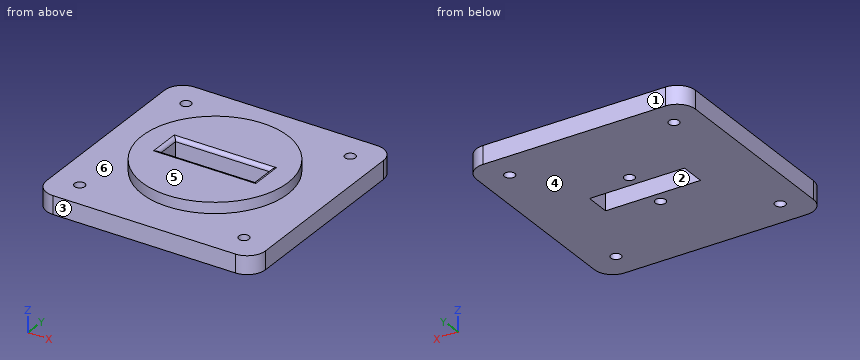
from build123d import *

# Parameters (mm, degrees)
F0_R     = 1.8034
F0_R_2   = 25.4
F0_W     = 33.02
F0_H     = 8.636
F1_DEPTH = 6.35
F2_R     = 25.4
F3_DEPTH = 3.81
F4_DEPTH = 12.7
F5_R     = 1.27


# Not quite as in the source:
# - a feature names something its author has since deleted; it is built from what else it names


with BuildPart() as f1:
    # F0 (on Top) → F1 (new body)
    with BuildSketch(Plane.XY):
        with BuildLine():
            Line((-31.75, -38.1), (31.75, -38.1))
            ThreePointArc((31.75, -38.1), (36.2401280605, -36.2401280605), (38.1, -31.75))
            Line((38.1, -31.75), (38.1, 31.75))
            ThreePointArc((38.1, 31.75), (36.2401280605, 36.2401280605), (31.75, 38.1))
            Line((31.75, 38.1), (-31.75, 38.1))
            ThreePointArc((-31.75, 38.1), (-36.2401280605, 36.2401280605), (-38.1, 31.75))
            Line((-38.1, 31.75), (-38.1, -31.75))
            ThreePointArc((-38.1, -31.75), (-36.2401280605, -36.2401280605), (-31.75, -38.1))
        make_face()
        with Locations((-28.575, -28.575)):
            Circle(F0_R, mode=Mode.SUBTRACT)
        with Locations((28.575, -28.575)):
            Circle(F0_R, mode=Mode.SUBTRACT)
        with Locations((-28.575, 28.575)):
            Circle(F0_R, mode=Mode.SUBTRACT)
        Circle(F0_R_2, mode=Mode.SUBTRACT)
        with Locations((28.575, 28.575)):
            Circle(F0_R, mode=Mode.SUBTRACT)
        Circle(F0_R_2)
        with Locations((0, -8.382)):
            Circle(F0_R, mode=Mode.SUBTRACT)
        Rectangle(F0_W, F0_H, mode=Mode.SUBTRACT)
        with Locations((0, 8.382)):
            Circle(F0_R, mode=Mode.SUBTRACT)
    extrude(amount=F1_DEPTH)

    # F2 (on face) → F3 (join)
    with BuildSketch(Plane.XY.offset(6.35)):
        Circle(F2_R)
    extrude(amount=F3_DEPTH)

    # F0 (on Top) → F4 (cut, symmetric)
    with BuildSketch(Plane.XY):
        Rectangle(F0_W, F0_H)
    extrude(amount=F4_DEPTH, both=True, mode=Mode.SUBTRACT)

    # F5
    f5_edges = [f1.edges().sort_by_distance(p)[0] for p in [
        (0, 4.318, 10.16),
        (-16.51, 0, 10.16),
        (0, -4.318, 10.16),
        (16.51, 0, 10.16),
    ]]
    fillet(f5_edges, radius=F5_R)


solid = f1.part
Here's how the part is built. I have some questions about the finished solid (model axes, mm). Face numbers are marked on the shaded views. A direction names the side the tool comes from. Coordinates: 2 decimals unless noted, no trailing zeros. Loops run counter-clockwise (first coordinate to the right, second up) from the corner with the lowest first, then second, coordinate; pieces in that order, holes last.
1. I need wall thicknesses on L1, parallel to Y at x = 0, z = 2.25; L2, parallel to X at y = 0.5, z = 4.75; L3, parallel to Y at x = 16, z = 5.75. Which ranges of each line are inside material? Lowest first, please.
2. Imagine slicing it at A-A, the plane y = 0. Please give me the cut outline in (x, z).
3. Imagine slicing it at C-C, the plane z = 1.25. Please give me the cut outline in (x, y) (3 decimals).
4. If we mould it in two halves opening along Y, with no side actions, what happens to the marked faces 1, 2, 3 and 4? For each: pulls with the +Y half, pulls with the -Y half, needs draft (parallel to the pull), parting line crosses it, or undercut.
5. For the marked faces 5 and 6, which set-ups out of +Z, -Z, +X, -X, +Y, -Y let a thin tool reach every point of the face, with its end or its side?
6. Imagine slicing it at D-D, the plane y = 14. Please give me the cut outline in (x, z), and give its area (3 significant figures).
7. Imagine slicing it at B-B, the plane x = 0. Please give me the cut outline in (y, z).
8. For P1, Ø1.1, axis at x = 0.5, y = 8.5, coming from the -Z side; P2, Ø4, axis at x = 28.575, y = -28.575, coming from the +Z side, each with a flat end and sliding along its axis, tell me the tip position at first contact or that it passes through.
Taken from the geometry:
1. L1: y = -38.1 to -10.19, -6.58 to -4.32, 4.32 to 6.58, 10.19 to 38.1
1. L2: x = -38.1 to -16.51, 16.51 to 38.1
1. L3: y = -38.1 to -4.32, 4.32 to 38.1
2. outline: (-38.1, 0) - (-16.51, 0) - (-16.51, 8.89) arc R1.27 ccw to (-17.78, 10.16) - (-25.4, 10.16) - (-25.4, 6.35) - (-38.1, 6.35) - close; (16.51, 0) - (38.1, 0) - (38.1, 6.35) - (25.4, 6.35) - (25.4, 10.16) - (17.78, 10.16) arc R1.27 ccw to (16.51, 8.89) - close
3. outline: (-38.1, -31.75) arc R6.35 ccw to (-31.75, -38.1) - (31.75, -38.1) arc R6.35 ccw to (38.1, -31.75) - (38.1, 31.75) arc R6.35 ccw to (31.75, 38.1) - (-31.75, 38.1) arc R6.35 ccw to (-38.1, 31.75) - close; hole circle Ø3.607 at (-28.575, -28.575); hole circle Ø3.607 at (-28.575, 28.575); hole (-16.51, -4.318) - (16.51, -4.318) - (16.51, 4.318) - (-16.51, 4.318) - close; hole circle Ø3.607 at (0, -8.382); hole circle Ø3.607 at (0, 8.382); hole circle Ø3.607 at (28.575, -28.575); hole circle Ø3.607 at (28.575, 28.575)
4. face 1: pulls with the +Y half
4. face 2: undercut
4. face 3: pulls with the -Y half
4. face 4: needs draft
5. face 5: +Z, +X, -X, +Y, -Y
5. face 6: +Z
6. outline: (-38.1, 0) - (38.1, 0) - (38.1, 6.35) - (21.19, 6.35) - (21.19, 10.16) - (-21.19, 10.16) - (-21.19, 6.35) - (-38.1, 6.35) - close
6. area: 645 mm2
7. outline: (-38.1, 0) - (-10.19, 0) - (-10.19, 6.35) - (-6.58, 6.35) - (-6.58, 0) - (-4.32, 0) - (-4.32, 8.89) arc R1.27 ccw to (-5.59, 10.16) - (-25.4, 10.16) - (-25.4, 6.35) - (-38.1, 6.35) - close; (4.32, 0) - (6.58, 0) - (6.58, 6.35) - (10.19, 6.35) - (10.19, 0) - (38.1, 0) - (38.1, 6.35) - (25.4, 6.35) - (25.4, 10.16) - (5.59, 10.16) arc R1.27 ccw to (4.32, 8.89) - close
8. P1: stops at z = 6.35
8. P2: stops at z = 6.35
